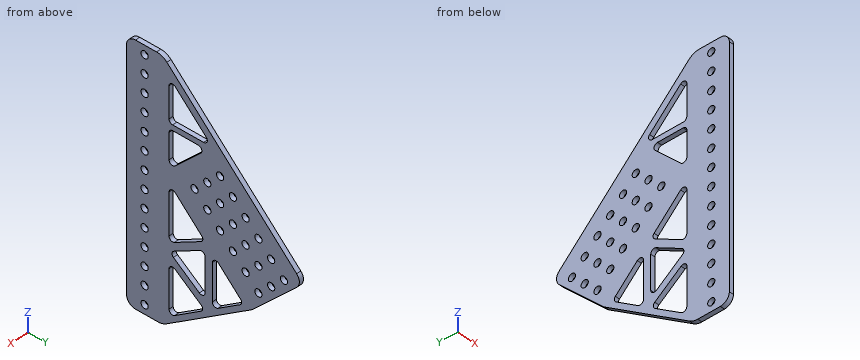
from build123d import *

# Parameters (mm, degrees)
SKETCH8_R           = 2.54
BOSS_EXTRUDE1_DEPTH = 3.175
FILLET1_R           = 2.54
FILLET2_R           = 6.35
FILLET3_R           = 10.16
FILLET4_R           = 12.7


with BuildPart() as part:
    # Sketch8 → Boss-Extrude1 (new body)
    with BuildSketch(Plane(origin=(0, 0, 0), x_dir=(0, 0, -1), z_dir=(1, 0, 0))):
        Polygon((181.332817332, 194.032817332), (217.253841816, 158.111792847), (260.35, 95.25), (260.35, 69.85), (82.55, 69.85), (82.55, 95.25), align=None)
        with Locations((185.822945392, 144.641408666)):
            Circle(SKETCH8_R, mode=Mode.SUBTRACT)
        with Locations((167.86243315, 162.601920908)):
            Circle(SKETCH8_R, mode=Mode.SUBTRACT)
        with Locations((167.86243315, 144.641408666)):
            Circle(SKETCH8_R, mode=Mode.SUBTRACT)
        with Locations((158.882177029, 135.661152545)):
            Circle(SKETCH8_R, mode=Mode.SUBTRACT)
        with Locations((158.882177029, 153.621664787)):
            Circle(SKETCH8_R, mode=Mode.SUBTRACT)
        with Locations((149.901920908, 144.641408666)):
            Circle(SKETCH8_R, mode=Mode.SUBTRACT)
        with Locations((140.921664787, 135.661152545)):
            Circle(SKETCH8_R, mode=Mode.SUBTRACT)
        with Locations((149.901920908, 126.680896424)):
            Circle(SKETCH8_R, mode=Mode.SUBTRACT)
        with Locations((158.882177029, 117.700640303)):
            Circle(SKETCH8_R, mode=Mode.SUBTRACT)
        with Locations((167.86243315, 126.680896424)):
            Circle(SKETCH8_R, mode=Mode.SUBTRACT)
        with Locations((176.842689271, 135.661152545)):
            Circle(SKETCH8_R, mode=Mode.SUBTRACT)
        with Locations((176.842689271, 153.621664787)):
            Circle(SKETCH8_R, mode=Mode.SUBTRACT)
        with Locations((194.803201513, 153.621664787)):
            Circle(SKETCH8_R, mode=Mode.SUBTRACT)
        with Locations((203.783457634, 162.601920908)):
            Circle(SKETCH8_R, mode=Mode.SUBTRACT)
        with Locations((194.803201513, 171.582177029)):
            Circle(SKETCH8_R, mode=Mode.SUBTRACT)
        with Locations((185.822945392, 180.56243315)):
            Circle(SKETCH8_R, mode=Mode.SUBTRACT)
        with Locations((176.842689271, 171.582177029)):
            Circle(SKETCH8_R, mode=Mode.SUBTRACT)
        with Locations((185.822945392, 162.601920908)):
            Circle(SKETCH8_R, mode=Mode.SUBTRACT)
        with Locations((254, 82.55)):
            Circle(SKETCH8_R, mode=Mode.SUBTRACT)
        with Locations((241.3, 82.55)):
            Circle(SKETCH8_R, mode=Mode.SUBTRACT)
        with Locations((228.6, 82.55)):
            Circle(SKETCH8_R, mode=Mode.SUBTRACT)
        with Locations((215.9, 82.55)):
            Circle(SKETCH8_R, mode=Mode.SUBTRACT)
        with Locations((203.2, 82.55)):
            Circle(SKETCH8_R, mode=Mode.SUBTRACT)
        with Locations((190.5, 82.55)):
            Circle(SKETCH8_R, mode=Mode.SUBTRACT)
        with Locations((177.8, 82.55)):
            Circle(SKETCH8_R, mode=Mode.SUBTRACT)
        with Locations((165.1, 82.55)):
            Circle(SKETCH8_R, mode=Mode.SUBTRACT)
        with Locations((152.4, 82.55)):
            Circle(SKETCH8_R, mode=Mode.SUBTRACT)
        with Locations((139.7, 82.55)):
            Circle(SKETCH8_R, mode=Mode.SUBTRACT)
        with Locations((127, 82.55)):
            Circle(SKETCH8_R, mode=Mode.SUBTRACT)
        with Locations((114.3, 82.55)):
            Circle(SKETCH8_R, mode=Mode.SUBTRACT)
        with Locations((101.6, 82.55)):
            Circle(SKETCH8_R, mode=Mode.SUBTRACT)
        with Locations((88.9, 82.55)):
            Circle(SKETCH8_R, mode=Mode.SUBTRACT)
        Polygon((164.270330702, 99.740128061), (203.862933209, 99.740128061), (189.670330702, 125.140128061), align=None, mode=Mode.SUBTRACT)
        Polygon((209.682177029, 99.740128061), (195.489574522, 125.140128061), (228.872016188, 125.140128061), align=None, mode=Mode.SUBTRACT)
        Polygon((216.048997042, 99.740128061), (252.652313741, 99.740128061), (235.238836201, 125.140128061), align=None, mode=Mode.SUBTRACT)
        Polygon((194.750330702, 130.220128061), (231.756140693, 130.220128061), (216.70480924, 152.174606599), align=None, mode=Mode.SUBTRACT)
        Polygon((124.757203769, 130.272998872), (94.224332957, 99.740128061), (124.757203769, 99.740128061), align=None, mode=Mode.SUBTRACT)
        Polygon((128.567203769, 126.462998872), (128.567203769, 99.740128061), (155.290074581, 99.740128061), align=None, mode=Mode.SUBTRACT)
    extrude(amount=BOSS_EXTRUDE1_DEPTH)

    # Fillet1
    fillet1_edges = [part.edges().sort_by_distance(p)[0] for p in [
        (1.5875, 125.140128061, -195.489574522),
        (1.5875, 99.740128061, -209.682177029),
        (1.5875, 125.140128061, -228.872016188),
        (1.5875, 99.740128061, -164.270330702),
        (1.5875, 99.740128061, -203.862933209),
        (1.5875, 125.140128061, -189.670330702),
        (1.5875, 99.740128061, -216.048997042),
        (1.5875, 99.740128061, -252.652313741),
        (1.5875, 125.140128061, -235.238836201),
        (1.5875, 130.220128061, -194.750330702),
        (1.5875, 130.220128061, -231.756140693),
        (1.5875, 152.174606599, -216.70480924),
        (1.5875, 130.272998872, -124.757203769),
        (1.5875, 99.740128061, -94.224332957),
        (1.5875, 99.740128061, -124.757203769),
        (1.5875, 126.462998872, -128.567203769),
        (1.5875, 99.740128061, -128.567203769),
        (1.5875, 99.740128061, -155.290074581),
    ]]
    fillet(fillet1_edges, radius=FILLET1_R)

    # Fillet2
    fillet2_edges = [part.edges().sort_by_distance(p)[0] for p in [
        (1.5875, 69.85, -260.35),
        (1.5875, 69.85, -82.55),
        (1.5875, 194.032817332, -181.332817332),
    ]]
    fillet(fillet2_edges, radius=FILLET2_R)

    # Fillet3
    fillet3_edges = [part.edges().sort_by_distance(p)[0] for p in [
        (1.5875, 95.25, -82.55),
        (1.5875, 95.25, -260.35),
    ]]
    fillet(fillet3_edges, radius=FILLET3_R)

    # Fillet4
    fillet4_edges = [part.edges().sort_by_distance(p)[0] for p in [
        (1.5875, 158.111792847, -217.253841816),
    ]]
    fillet(fillet4_edges, radius=FILLET4_R)


solid = part.part
Design review of the part built by this model. Coordinates are the model's own, in mm. Coordinates: 2 decimals unless noted, no trailing zeros. Use a Markdown table: item, result.
(1) Add section A-A (x = 2.3). Count the separate pieces of the cut face and the enclosed holes in it, then the cut area to 3 significant figures.
Worked answers:
| item | result |
|---|---|
| separate pieces | 1 |
| enclosed holes | 38 |
| area | 10,400 mm2 |
(2) Wall thickness on probe 1 along Y at (x, z) = (2.65, -184); probe 2 along Y at (x, z) = (2.75, -191); probe 3 along Y at (x, z) = (1.45, -166): over which ranges is each line inside the solid? List them lowest first.
Worked answers:
| item | result |
|---|---|
| probe 1 | y = 69.85 to 99.74, 119.47 to 142.87, 146.41 to 160.83, 164.37 to 178.79, 182.33 to 190.82 |
| probe 2 | y = 69.85 to 80.06, 85.04 to 99.74, 122.64 to 184.37 |
| probe 3 | y = 69.85 to 80.17, 84.93 to 124.95, 128.41 to 142.91, 146.37 to 160.87, 164.33 to 178.7 |
(3) For P1, Ø1.6, axis at x = 1, z = -143.5, coming from the +Y side; P2, Ø1.5, axis at x = 1.5, y = 148, coming from the -Z side; P3, Ø1, axis at x = 1, z = -209.5, coming from the +Y side, all flat-tipped, find the tip position at first contact; note any pin that passes through.
Worked answers:
| item | result |
|---|---|
| P1 | stops at y = 157 |
| P2 | stops at z = -224.7 |
| P3 | stops at y = 166.37 |
